Autodesk Inventor part; units mm, degrees
ref_plane "Work Plane1" through (11.4164, 0, 0) normal (0, 0, 1) x (-1, 0, 0)
ref_plane "YZ Plane" through (0, 0, 0) normal (1, 0, 0) x (0, 1, 0)
ref_plane "XZ Plane" through (0, 0, 0) normal (0, 1, 0) x (-1, 0, 0)
sketch "Sketch1" plane through (0, 0, 0) normal (1, 0, 0) x (0, 1, 0)
  line L0 (-4.0415, 0) -> (-2.0207, 3.5)
  line L1 (-2.0207, 3.5) -> (2.0207, 3.5)
  line L2 (2.0207, 3.5) -> (4.0415, 0)
  line L3 (4.0415, 0) -> (2.0207, -3.5)
  line L4 (2.0207, -3.5) -> (-2.0207, -3.5)
  line L5 (-2.0207, -3.5) -> (-4.0415, 0)
  point P0 (0, 0)
  point P1 (0, 0)
  dimension "d0" = 8.0829
extrude "Body" add sketch "Sketch1" along normal blind 4
sketch "Sketch2" plane through (0, 0, 0) normal (-1, 0, 0) x (0, 0, 1)
  line L0 (0, -5.658) -> (0, 5.658)
  line L1 (-4.9, 0) -> (4.9, 0)
  point P0 (0, 0)
hole "Thread" at (0, 0, 0) direction (1, 0, 0) diameter 3.242 end through all
chamfer "Chamfer1" distance 0.3789 angle 30 1 edges at (0, 0, -1.621) measured on face at (0, -2.4654, -1.4736)
chamfer "Chamfer2" distance 0.3789 angle 30 1 edges at (4, 0, -1.621) measured on face at (4, -2.4654, -1.4736)
sketch "Sketch3" plane through (0, 0, 0) normal (0, 0, 1) x (1, 0, 0)
  line L0 (0, 2.0207) -> (0, 4.0415)
  line L1 (0, 4.0415) -> (4, 4.0415)
  line L2 (4, 2.0207) -> (4, 4.0415)
  line L3 (-0.8, 0) -> (4.8, 0)
  line L4 (0.3126, 4.0415) -> (0, 3.5)
  line L5 (4, 2.975) -> (3.1709, 2.975)
  line L6 (3.1709, 2.975) -> (1.9, 4.0415)
  dimension "d3" = 30
  dimension "d5" = 7
  dimension "d6" = 5.95
  dimension "d8" = 50
  dimension "d9" = 1.9
revolve "Chamfer3" cut sketch "Sketch3" angle 360 about axis through (-10, 0, 0) along (1, 0, 0)
ref_plane "Work Plane1" through (11.4164, 0, 0) normal (0, 0, 1) x (-1, 0, 0)
equation "\"d0\" = 1.1547 * SW"
equation "\"d1\" = KOH"
equation "\"d3\" = ANG1"
equation "\"d5\" = SW0"
equation "\"d6\" = SW1"
equation "\"d8\" = ANG2"
equation "\"d9\" = KOH1"
equation "\"d10\" = -0.5 * GD1 + 0.5 * NND"
equation "\"d39\" = -0.5 * GD1 + 0.5 * NND"
equation "\"d12\" = -0.5 * GD1 + 0.5 * NND"
equation "\"d40\" = -0.5 * GD1 + 0.5 * NND"
equation "\"ANG1\" = 30deg"
equation "\"ANG2\" = 50deg"
equation "\"NND\" = 4"
equation "\"KOH\" = 4"
equation "\"SW\" = 7"
equation "\"SW0\" = SW"
equation "\"SW1\" = 0.85 * SW"
equation "\"KOH1\" = 1.9"
equation "\"GUL\" = 0.541266 * PTC"
equation "\"THREADDIA\" = 4"
equation "\"TOA\" = 30deg"
equation "\"PTC\" = 0.7"
equation "\"E0\" = 1.155 * SW"
equation "\"GAL\" = 0.541266 * PTC"
properties part number "ANSI B18.16.3M - Property Class 9 - Metric M4 x 0.7 Metal Type" material "Steel, Mild"
Read the model definition and answer for the solid it produces. Units are mm, in the model's axes. A direction names the side the tool comes from. Give positions to 0.01 mm unless a question says otherwise; leave off trailing zeros. Write each loop counter-clockwise with the first axis right and the second up, starting at its lowest first coordinate (ties: lowest second). Pieces come first, ordered by that corner, then holes. Notation, with made-up numbers: (12.5, -18) - (43.5, -18) arc R17 cw to (43.5, 5) - close; hole circle Ø1 at (81.5, -14). An arc over 180 degrees is marked (long way). Answer in a Markdown table with one row per item. Add a question column.
Item 1: Section C-C, the plane x = 2.75 is taken. Write down the section's boundary in (y, z), and give its area (3 significant figures).
Item 2: Flat-ended cylindrical pins translate along their axes: P1, Ø1, axis at x = 1, z = -1.5, coming from the +Y side; P2, Ø1.5, axis at x = 3, z = 0.5, coming from the -Y side; P3, Ø3.5, axis at y = 0, z = 0, coming from the -X side. Find the tip coordinate at first contact, or state that the pin passes through.
Item 3: A tool of negligible diameter and unlimited length cuts with its end or side. For faces 4 (the face through (3.6, -2.2, -2)), 5 (the face through (1.3, -3, -1.8)), from which of +Z, -Z, +X, -X, +Y, -Y can it reach the whole face along a straight path? Write none if from no direction.
Item 4: Section A-A, the plane x = 1.1 is taken. Write down the section's boundary in (y, z).
Item 5: Determine the mould class of faces 1 (the face through (1, 0, 3.5)), 2 (the face through (2.025, 1.438, 0.748)), 3 (the face through (0.076, -1.808, 3.15)) for opening direction Y: pulls with the +Y half, pulls with the -Y half, needs draft (parallel to the pull), parting line crosses it, or undercut.
Item 6: Section B-B, the plane x = 3.45 is taken. Write down the section's boundary in (y, z) (3 decimals), and give its area (3 significant figures).
Item 7: Find the intervals of material crossed by L1, parallel to Z at x = 1.65, y = 0; L2, parallel to Z at x = 3.3, y = 0 (3 decimals); L3, parallel to Y at x = 2.15, z = 0, in increasing order.
Recorded:
| question | item | result |
|---|---|---|
| 1 | outline | circle Ø6.66 at (0, 0); hole circle Ø3.24 at (0, 0) |
| 1 | area | 26.5 mm2 |
| 2 | P1 | stops at y = 3.46 |
| 2 | P2 | stops at y = -3.72 |
| 2 | P3 | stops at x = 0.14 |
| 3 | face 4 | +X |
| 3 | face 5 | -Z, +X, -X, -Y |
| 4 | outline | (-4.04, 0) - (-2.02, -3.5) - (2.02, -3.5) - (4.04, 0) - (2.02, 3.5) - (-2.02, 3.5) - close; hole circle Ø3.24 at (0, 0) |
| 5 | face 1 | needs draft |
| 5 | face 2 | undercut |
| 5 | face 3 | pulls with the -Y half |
| 6 | outline | circle Ø5.95 at (0, 0); hole circle Ø3.242 at (0, 0) |
| 6 | area | 19.6 mm2 |
| 7 | L1 | z = -3.5 to -1.62, 1.62 to 3.5 |
| 7 | L2 | z = -2.975 to -1.621, 1.621 to 2.975 |
| 7 | L3 | y = -3.83 to -1.62, 1.62 to 3.83 |
